The listing builds one solid part. Answer for the finished solid, in the listing's coordinates (mm). Face numbers are marked on the shaded views. A direction names the side the tool comes from. Coordinates: 2 decimals unless noted, no trailing zeros. Loops run counter-clockwise (first coordinate to the right, second up) from the corner with the lowest first, then second, coordinate; pieces in that order, holes last. Notation, with made-up numbers: (-15.5, 39) - (20.5, 39) arc R26 ccw to (20.5, 62) - close; hole circle Ø1 at (17.25, 79.5). An arc over 180 degrees is marked (long way). Write each question's results on one line, items separated by ' | '. Start each with the question number.
(1) Determine the mould class of the marked faces 3, 4 and 5 for opening direction Y: released by +Y, released by -Y, zero draft, split by the parting line, or undercut.
(2) Find section D-D on y = 508. Determine the outline of the cut face in (x, z), then the cut area to 3 significant figures.
(3) Find section A-A on x = 633.5. Determine the outline of the cut face in (y, z).
(4) Find section C-C on z = 586. Determine the outline of the cut face in (x, y).
(5) For the marked faces 1 and 2, determine the directions among +Z, -Z, +X, -X, +Y, -Y from which every point of the face is accessible in a straight line to the end or side of a thin tool.
(6) Consider line 1 (Y direction, x = 381.5, z = 650); line 2 (Z direction, x = 406.4, y = 945.5); line 3 (X direction, y = 859, z = 413.5). Determine where each line is inside the solid, lowest interval first. Write a range as from..to.
(7) Given pin 1 Ø3 at (y, z) = (836, 183.5) entering from +X; pin 2 Ø6 at (x, z) = (731.5, 141.5) entering from -Y; pin 3 Ø10 at (y, z) = (163.5, 727) entering from -X, each flat-ended and moving along its own axis, determine where each tip first touches the part or whether it passes through.
from build123d import *

# Parameters (mm, degrees)
F1_DEPTH = 812.8
F2_R     = 406.39999
F3_R     = 203.2
F4_DEPTH = 1016.001
F5_R     = 203.2
F6_DEPTH = 812.8


# Not quite as in the source:
# - a fillet or chamfer is up to 0.001 mm smaller than in the source, because OpenCascade refuses the exact size


with BuildPart() as f1:
    # F0 (on Top) → F1 (new body)
    with BuildSketch(Plane.XY):
        Polygon((0, 279.4), (0, 0), (1320.8, 0), (1320.8, 1016), (0, 1016), (0, 736.6), (1041.4, 736.6), (1041.4, 279.4), align=None)
    extrude(amount=F1_DEPTH)

    # F2 (radius 406.4 in the source; OpenCascade refuses exactly that, so slightly less here)
    f2_edges = [f1.edges().sort_by_distance(p)[0] for p in [
        (0, 139.7, 812.8),
        (0, 139.7, 0),
        (0, 876.3, 0),
        (0, 876.3, 812.8),
    ]]
    fillet(f2_edges, radius=F2_R)

    # F3 (on face) → F4 (cut, through all)
    with BuildSketch(Plane.XZ):
        with Locations((406.4, 406.4)):
            Circle(F3_R)
    extrude(amount=-F4_DEPTH, mode=Mode.SUBTRACT)

    # F5 (on face) → F6 (join)
    with BuildSketch(Plane.YZ.offset(1320.8)):
        with Locations((508, 406.4)):
            Circle(F5_R)
    extrude(amount=F6_DEPTH)


solid = f1.part
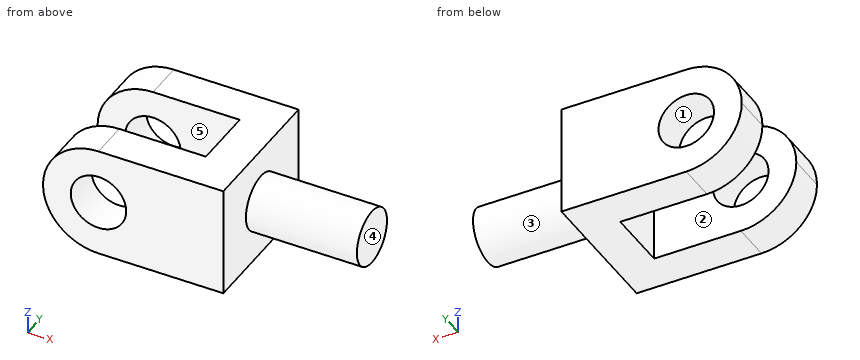
Values:
1) face 3: split by the parting line | face 4: zero draft | face 5: undercut
2) outline: (1041.4, 0) - (1320.8, 0) - (1320.8, 203.2) - (2133.6, 203.2) - (2133.6, 609.6) - (1320.8, 609.6) - (1320.8, 812.8) - (1041.4, 812.8) - close | area: 557,000 mm²
3) outline: (0, 0) - (279.4, 0) - (279.4, 812.8) - (0, 812.8) - close; (736.6, 0) - (1016, 0) - (1016, 812.8) - (736.6, 812.8) - close
4) outline: (41.84, 0) - (311.35, 0) - (311.35, 279.4) - (41.84, 279.4) - close; (41.84, 736.6) - (311.35, 736.6) - (311.35, 1016) - (41.84, 1016) - close; (501.45, 0) - (1320.8, 0) - (1320.8, 412.95) - (2133.6, 412.95) - (2133.6, 603.05) - (1320.8, 603.05) - (1320.8, 1016) - (501.45, 1016) - (501.45, 736.6) - (1041.4, 736.6) - (1041.4, 279.4) - (501.45, 279.4) - close
5) face 1: +Y, -Y | face 2: +Z, -Z, -X
6) line 1: y = 0..279.4, 736.6..1016 | line 2: z = 0..203.2, 609.6..812.8 | line 3: x = 0.06..203.32, 609.48..1320.8
7) pin 1: stops at x = 1320.8 | pin 2: stops at y = 0 | pin 3: stops at x = 150.36
